Input: part model. Units: mm. Frame: model coordinates. A direction names the side the tool comes from. Coordinates: 2 decimals unless noted, no trailing zeros. Order: outer loops, then holes, each group sorted by start corner. A loop starts at its lowest first (then second) coordinate and runs counter-clockwise, first axis right, second up. Notation, with made-up numbers: (37.25, -36) -> (47.25, -36) arc R8 cw to (47.25, -31) -> close; hole circle Ø4 at (61.5, 21). An arc over 180 degrees is marked (long way). Write each question's results on one line, items separated by ' | '.
```python
from build123d import *

# Parameters (mm, degrees)
BOSS_EXTRUDE1_DEPTH = 4
BOSS_EXTRUDE2_START = -5
SKETCH1_4_R         = 0.95
BOSS_EXTRUDE2_DEPTH = 5
CHAMFER1_SIZE       = 0.4


with BuildPart() as part:
    # Sketch1 → Boss-Extrude1 (new body)
    with BuildSketch(Plane.XY):
        with BuildLine():
            Line((11.4, 0.95), (0, 0.95))
            ThreePointArc((0, 0.95), (-0.95, 0), (0, -0.95))
            Line((0, -0.95), (11.4, -0.95))
            ThreePointArc((11.4, -0.95), (12.35, 0), (11.4, 0.95))
        make_face()
    extrude(amount=BOSS_EXTRUDE1_DEPTH)

    # Sketch1<4> → Boss-Extrude2 (add)
    with BuildSketch(Plane.XY.offset(BOSS_EXTRUDE2_START)):
        with Locations(Location((0, 0, 0), (0, 0, 90))):
            Circle(SKETCH1_4_R)
        with Locations(Location((11.4, 0, 0), (0, 0, 270))):
            Circle(SKETCH1_4_R)
    extrude(amount=BOSS_EXTRUDE2_DEPTH)

    # Chamfer1
    chamfer1_edges = [part.edges().sort_by_distance(p)[0] for p in [
        (0, -0.95, -5),
        (11.4, 0.95, -5),
    ]]
    chamfer(chamfer1_edges, length=CHAMFER1_SIZE)


solid = part.part
```
(1) Cut plane C-C, the plane z = 3.25. Return loops of the section in (x, y), plus the area to 3 significant figures.
Return value:
outline: (0, -0.95) -> (11.4, -0.95) arc R0.95 ccw to (11.4, 0.95) -> (0, 0.95) arc R0.95 ccw to start | area: 24.5 mm2
(2) Line query: line 1 along Z through (x, y) = (5.5, -0.25); line 2 along X through (y, z) = (-0.05, -3); line 3 along X through (y, z) = (0.7, -0.25). Output: solid intervals per line, ascending. Write a range as from..to.
Return value:
line 1: 0..4 | line 2: -0.95..0.95, 10.45..12.35 | line 3: -0.64..0.64, 10.76..12.04
(3) Mould query, pull axis X, two halves, no side actions, for faces 3 (the face through (11, 0, -5)), 4 (the face through (6, 0, 0)). Classes: +X half, -X half, draft (parallel to the pull), parting line (faces both ways), or undercut.
Return value:
face 3: draft | face 4: undercut
(4) Cut plane B-B, the plane y = 0. Return loops of the section in (x, z), plus the area to 3 significant figures.
Return value:
outline: (-0.95, -4.6) -> (-0.55, -5) -> (0.55, -5) -> (0.95, -4.6) -> (0.95, 0) -> (10.45, 0) -> (10.45, -4.6) -> (10.85, -5) -> (11.95, -5) -> (12.35, -4.6) -> (12.35, 4) -> (-0.95, 4) -> close | area: 71.9 mm2
(5) Cut plane D-D, the plane x = 7.25. Return loops of the section in (y, z).
Return value:
outline: (-0.95, 0) -> (0.95, 0) -> (0.95, 4) -> (-0.95, 4) -> close
(6) Pin query (flat end, axial travel): P1, Ø1, axis at x = 5, y = 0, coming from the -Z side. Return the tip coordinate at first contact, or that it passes through.
Return value:
P1: z = 0
(7) Cut plane A-A, the plane z = -4. Return loops of the section in (x, y), plus the area to 3 significant figures.
Return value:
outline: circle Ø1.9 at (0, 0); circle Ø1.9 at (11.4, 0) | area: 5.67 mm2
(8) Reachability of faces 1 (the face through (12.342, 0.124, -1.316)), 2 (the face through (6, -0.95, 2)) from +Z, -Z, +X, -X, +Y, -Y: full face, straight path, thin tool, end or side. Return the list, or none.
Return value:
face 1: -Z | face 2: +Z, -Z, +X, -X, -Y
